Verification items for the finished model (mm, model axes). Face numbers are marked on the shaded views. A direction names the side the tool comes from. Give positions to 0.01 mm unless a question says otherwise; leave off trailing zeros. Loops run counter-clockwise (first coordinate to the right, second up) from the corner with the lowest first, then second, coordinate; pieces in that order, holes last. Notation, with made-up numbers: M 9,16 L 38,16 A23 cw 38,51 Z; hole C 75,5 d7. An arc over 180 degrees is marked long. Use CSV: the item, a comma, the result in double quotes.
from build123d import *

# Parameters (mm, degrees)
F3_R       = 1.5
F4_DEPTH   = 27
F5_R       = 1.2
F6_DEPTH   = 8
F3_R_2     = 2.75
F4_FACE1_R = 1.5
F7_DEPTH   = 3
F8_SIZE    = 0.29999
F10_DEPTH  = 1.3


# Not quite as in the source:
# - a fillet or chamfer is up to 0.001 mm smaller than in the source, because OpenCascade refuses the exact size


with BuildPart() as f4:
    # F3 (on Top) → F4 (new body)
    with BuildSketch(Plane.XY):
        Circle(F3_R)
    extrude(amount=-F4_DEPTH)

    # F5 (on face) → F6 (join)
    with BuildSketch(Plane(origin=(0, 0, -27), x_dir=(1, 0, 0), z_dir=(0, 0, -1))):
        Circle(F5_R)
    extrude(amount=F6_DEPTH)

    # F3 (on Top) + F4_face1 (on face) → F7 (join)
    with BuildSketch(Plane.XY):
        Circle(F3_R_2)
        Circle(F3_R, mode=Mode.SUBTRACT)
    with BuildSketch(Plane.XY):
        Circle(F4_FACE1_R)
    extrude(amount=F7_DEPTH)

    # F8 (size 0.3 in the source; OpenCascade refuses exactly that, so slightly less here)
    f8_edges = [f4.edges().sort_by_distance(p)[0] for p in [
        (-1.5, 0, -27),
        (-2.75, 0, 3),
        (-1.2, 0, -35),
    ]]
    chamfer(f8_edges, length=F8_SIZE)

    # F9 (on face) → F10 (cut)
    with BuildSketch(Plane.XY.offset(3)):
        Polygon((1.25, -0.7216878365), (1.25, 0.7216878365), (0, 1.443375673), (-1.25, 0.7216878365), (-1.25, -0.7216878365), (0, -1.443375673), align=None)
    extrude(amount=-F10_DEPTH, mode=Mode.SUBTRACT)


solid = f4.part
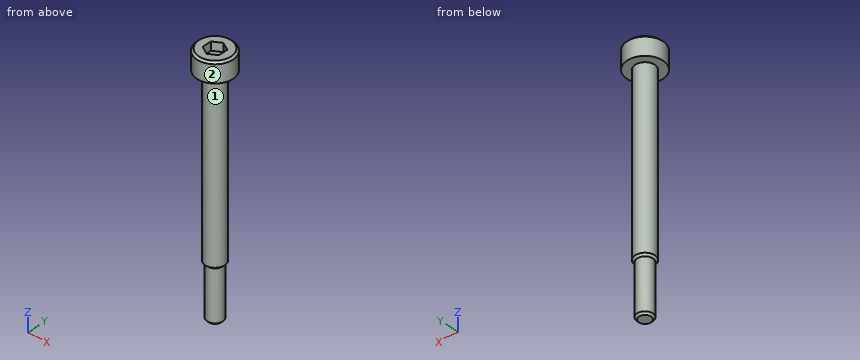
(1) Depth check by flat-ended pin: pin 1 Ø3 at (x, z) = (2, -9.5) entering from +Y; pin 2 Ø2 at (y, z) = (-1.5, -27.5) entering from +X; pin 3 Ø0.8 at (x, y) = (0, 0) entering from +Z. Enter the tip coordinate at first touch or a pass-through.
Calculated:
pin 1,"stops at y = 1.41"
pin 2,"stops at x = 1.2"
pin 3,"stops at z = 1.7"
(2) Section check B-B on z = -17. Record the cut outline in (x, y).
Calculated:
outline,"C 0,0 d3"
(3) Tool access check on the marked faces 1 and 2. Record the directions out of +Z, -Z, +X, -X, +Y, -Y that give a thin tool (end or side, any length) a straight path to the whole face; none if there is none.
Calculated:
face 1,"-Z"
face 2,"+Z, -Z"
(4) Scan lines: L1, parallel to Y at x = 0.1, z = -25.5; L2, parallel to Z at x = -1.2, y = -1.9; L3, parallel to Z at x = -0.4, y = -0.25. Record each from-to range of solid material in increasing order. Write a range as from..to.
Calculated:
L1,"y = -1.5..1.5"
L2,"z = 0..3"
L3,"z = -35..1.7"
